```python
from build123d import *

# Parameters (mm, degrees)
EXTRU_MINCE1_DEPTH      = 30
BOSS_EXTRU_1_DEPTH      = 2
ENL_V_MAT_EXTRU_1_DEPTH = 3
ESQUISSE3_R             = 2.5
BOSS_EXTRU_2_DEPTH      = 8
ESQUISSE4_R             = 1.25
BOSS_EXTRU_3_DEPTH      = 3


with BuildPart() as part:
    # Esquisse1 → Extru.-Mince1 (new body)
    with BuildSketch(Plane.XY):
        with BuildLine():
            Line((42.160194175, -58.330097087), (-32.839805825, -58.330097087))
            ThreePointArc((-32.839805825, -58.330097087), (-35.314679559, -57.304970822), (-36.339805825, -54.830097087))
            Line((-36.339805825, -54.830097087), (-36.339805825, 15.169902913))
            ThreePointArc((-36.339805825, 15.169902913), (-35.314679559, 17.644776647), (-32.839805825, 18.669902913))
            Line((-32.839805825, 18.669902913), (42.160194175, 18.669902913))
            ThreePointArc((42.160194175, 18.669902913), (44.635067909, 17.644776647), (45.660194175, 15.169902913))
            Line((45.660194175, 15.169902913), (45.660194175, -54.830097087))
            ThreePointArc((45.660194175, -54.830097087), (44.635067909, -57.304970822), (42.160194175, -58.330097087))
        make_face()
        with BuildLine():
            Line((42.160194175, -56.330097087), (-32.839805825, -56.330097087))
            ThreePointArc((-32.839805825, -56.330097087), (-33.900465997, -55.890757259), (-34.339805825, -54.830097087))
            Line((-34.339805825, -54.830097087), (-34.339805825, 15.169902913))
            ThreePointArc((-34.339805825, 15.169902913), (-33.900465997, 16.230563084), (-32.839805825, 16.669902913))
            Line((-32.839805825, 16.669902913), (42.160194175, 16.669902913))
            ThreePointArc((42.160194175, 16.669902913), (43.220854347, 16.230563084), (43.660194175, 15.169902913))
            Line((43.660194175, 15.169902913), (43.660194175, -54.830097087))
            ThreePointArc((43.660194175, -54.830097087), (43.220854347, -55.890757259), (42.160194175, -56.330097087))
        make_face(mode=Mode.SUBTRACT)
    extrude(amount=EXTRU_MINCE1_DEPTH)

    # Esquisse1<2> → Boss.-Extru.1 (add)
    with BuildSketch(Plane.XY):
        with BuildLine():
            Line((-32.839805825, 17.669902913), (42.160194175, 17.669902913))
            ThreePointArc((42.160194175, 17.669902913), (43.927961128, 16.937669866), (44.660194175, 15.169902913))
            Line((44.660194175, 15.169902913), (44.660194175, -54.830097087))
            ThreePointArc((44.660194175, -54.830097087), (43.927961128, -56.59786404), (42.160194175, -57.330097087))
            Line((42.160194175, -57.330097087), (-32.839805825, -57.330097087))
            ThreePointArc((-32.839805825, -57.330097087), (-34.607572778, -56.59786404), (-35.339805825, -54.830097087))
            Line((-35.339805825, -54.830097087), (-35.339805825, 15.169902913))
            ThreePointArc((-35.339805825, 15.169902913), (-34.607572778, 16.937669866), (-32.839805825, 17.669902913))
        make_face()
    extrude(amount=BOSS_EXTRU_1_DEPTH)

    # Esquisse2 → Enlèv. mat.-Extru.1 (cut)
    with BuildSketch(Plane.XY.offset(30)):
        with BuildLine():
            Line((-32.839805825, 17.669902913), (42.360194175, 17.669902913))
            ThreePointArc((42.360194175, 17.669902913), (44.127961128, 16.937669866), (44.860194175, 15.169902913))
            Line((44.860194175, 15.169902913), (44.860194175, -55.030097087))
            ThreePointArc((44.860194175, -55.030097087), (44.127961128, -56.79786404), (42.360194175, -57.530097087))
            Line((42.360194175, -57.530097087), (-32.839805825, -57.530097087))
            ThreePointArc((-32.839805825, -57.530097087), (-34.607572778, -56.79786404), (-35.339805825, -55.030097087))
            Line((-35.339805825, -55.030097087), (-35.339805825, 15.169902913))
            ThreePointArc((-35.339805825, 15.169902913), (-34.607572778, 16.937669866), (-32.839805825, 17.669902913))
        make_face()
    extrude(amount=-ENL_V_MAT_EXTRU_1_DEPTH, mode=Mode.SUBTRACT)

    # Esquisse3 → Boss.-Extru.2 (add)
    with BuildSketch(Plane.XY.offset(2)):
        with Locations((-20.339805825, 7.669902913)):
            Circle(ESQUISSE3_R)
        with Locations((29.860194175, 7.669902913)):
            Circle(ESQUISSE3_R)
        with Locations((29.860194175, -47.530097087)):
            Circle(ESQUISSE3_R)
        with Locations((-20.339805825, -47.530097087)):
            Circle(ESQUISSE3_R)
    extrude(amount=BOSS_EXTRU_2_DEPTH)

    # Esquisse4 → Boss.-Extru.3 (add)
    with BuildSketch(Plane.XY.offset(10)):
        with Locations((-20.339805825, 7.669902913)):
            Circle(ESQUISSE4_R)
        with Locations((29.860194175, 7.669902913)):
            Circle(ESQUISSE4_R)
        with Locations((-20.339805825, -47.530097087)):
            Circle(ESQUISSE4_R)
        with Locations((29.660194175, -47.330097087)):
            Circle(ESQUISSE4_R)
    extrude(amount=BOSS_EXTRU_3_DEPTH)


solid = part.part
```
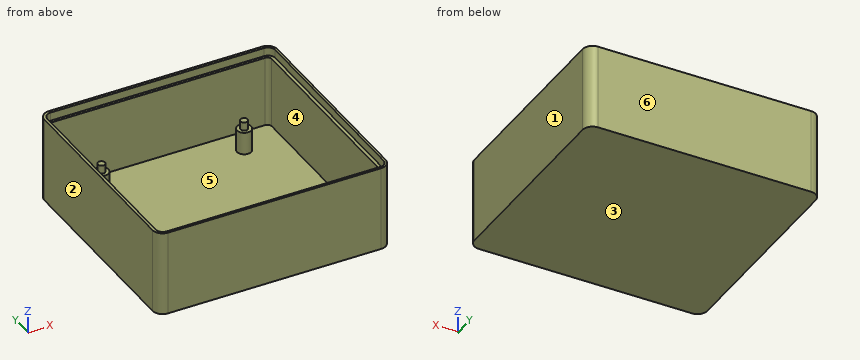
Geometry: final body of the model. Coordinates: model frame, mm. Face numbers are marked on the shaded views. A direction names the side the tool comes from. Coordinates: 2 decimals unless noted, no trailing zeros. Order: outer loops, then holes, each group sorted by start corner. A loop starts at its lowest first (then second) coordinate and runs counter-clockwise, first axis right, second up. Notation, with made-up numbers: M 75,83.5 L 99,83.5 A12 ccw 99,89.5 Z; hole C -17.5,35.5 d6. An arc over 180 degrees is marked long. Answer in a Markdown table with one row per item. Add a question column.
Q1. Section query B-B on x = -16.5. Return the cut outline in (y, z).
Q2. Reachability of the marked faces 5 and 6 from +Z, -Z, +X, -X, +Y, -Y: full face, straight path, thin tool, end or side. Return the list, or none.
Q3. Section query C-C on y = -21.5. Return the cut outline in (x, z), and give its area (3 significant figures).
Q4. Contact query for a flat-ended pin moving along its axis: P1, Ø1.2, axis at x = -20, y = -48, coming from the +Z side. Output: stop coordinate, or through.
Q5. Line query: L1, parallel to X at y = -24, z = 10.25; L2, parallel to Y at x = -31.5, z = 19.5; L3, parallel to X at y = -48.5, z = 4. Output: solid intervals per line, ascending.
Q6. Section query A-A on z = 12. Return the cut outline in (x, y).
Q7. Section query D-D on z = 21. Return the cut outline in (x, y), and give its area (3 significant figures).
Q8. Mould query, pull axis X, two halves, no side actions, for the marked faces 1, 2, 3 and 4. Classes: released by +X, released by -X, zero draft, split by the parting line, or undercut.
Completed:
| question | item | result |
|---|---|---|
| 1 | outline | M -58.33,0 L 18.67,0 L 18.67,30 L 17.67,30 L 17.67,27 L 16.67,27 L 16.67,2 L -56.33,2 L -56.33,27 L -57.53,27 L -57.53,30 L -58.33,30 Z |
| 2 | face 5 | +Z |
| 2 | face 6 | +Z, -Z, +X, -X, +Y |
| 3 | outline | M -36.34,0 L 45.66,0 L 45.66,30 L 44.86,30 L 44.86,27 L 43.66,27 L 43.66,2 L -34.34,2 L -34.34,27 L -35.34,27 L -35.34,30 L -36.34,30 Z |
| 3 | area | 269 mm2 |
| 4 | P1 | stops at z = 13 |
| 5 | L1 | x = -36.34 to -34.34, 43.66 to 45.66 |
| 5 | L2 | y = -58.33 to -56.33, 16.67 to 18.67 |
| 5 | L3 | x = -36.34 to -34.34, -22.64 to -18.04, 27.56 to 32.16, 43.66 to 45.66 |
| 6 | outline | M -36.34,-54.83 A3.5 ccw -32.84,-58.33 L 42.16,-58.33 A3.5 ccw 45.66,-54.83 L 45.66,15.17 A3.5 ccw 42.16,18.67 L -32.84,18.67 A3.5 ccw -36.34,15.17 Z; C -20.34,-47.53 d2.5; C -20.34,7.67 d2.5; C 29.66,-47.33 d2.5; C 29.86,7.67 d2.5; hole M -34.34,-54.83 A1.5 ccw -32.84,-56.33 L 42.16,-56.33 A1.5 ccw 43.66,-54.83 L 43.66,15.17 A1.5 ccw 42.16,16.67 L -32.84,16.67 A1.5 ccw -34.34,15.17 Z |
| 7 | outline | M -36.34,-54.83 A3.5 ccw -32.84,-58.33 L 42.16,-58.33 A3.5 ccw 45.66,-54.83 L 45.66,15.17 A3.5 ccw 42.16,18.67 L -32.84,18.67 A3.5 ccw -36.34,15.17 Z; hole M -34.34,-54.83 A1.5 ccw -32.84,-56.33 L 42.16,-56.33 A1.5 ccw 43.66,-54.83 L 43.66,15.17 A1.5 ccw 42.16,16.67 L -32.84,16.67 A1.5 ccw -34.34,15.17 Z |
| 7 | area | 611 mm2 |
| 8 | face 1 | released by +X |
| 8 | face 2 | released by -X |
| 8 | face 3 | zero draft |
| 8 | face 4 | undercut |
